Autodesk Inventor part; units mm, degrees
ref_plane "YZ Plane" through (0, 0, 0) normal (1, 0, 0) x (0, 1, 0)
ref_plane "XZ Plane" through (0, 0, 0) normal (0, 1, 0) x (-1, 0, 0)
ref_plane "XY Plane" through (0, 0, 0) normal (0, 0, 1) x (1, 0, 0)
sketch "Sketch1" plane through (0, 0, 0) normal (0, 1, 0) x (-1, 0, 0)
  line L0 (-9.525, -13.4747) -> (9.525, -13.4747)
  line L1 (9.525, -13.4747) -> (9.525, 13.4747)
  line L2 (9.525, 13.4747) -> (-9.525, 13.4747)
  line L3 (-9.525, 13.4747) -> (-9.525, -13.4747)
  line L4 (-9.525, -13.4747) -> (9.525, 13.4747) construction
  line L5 (9.525, -13.4747) -> (-9.525, 13.4747) construction
  point P0 (0, 0)
  dimension "d0" = 19.05
  dimension "d1" = 26.9494
extrude "Extrusion1" add sketch "Sketch1" along normal blind 26.9494
sketch "Sketch2" plane through (9.525, 0, 13.4747) normal (1, 0, 0) x (0, 0, -1)
  line L0 (26.9494, 26.9494) -> (0, 26.9494)
  line L1 (0, 26.9494) -> (26.9494, 0)
  line L2 (0, 0) -> (26.9494, 0)
  line L3 (26.9494, 0) -> (26.9494, 26.9494)
  line L4 (0, 26.9494) -> (26.9494, 26.9494)
  line L5 (0, 0) -> (0, 26.9494)
  point P0 (13.4747, 0)
extrude "Extrusion2" cut sketch "Sketch2" against normal blind 19.05 contours L3 L1 L0
sketch "Sketch3" plane through (0, 0, 0) normal (0, -1, 0) x (1, 0, 0)
  circle A0 centre (0, 0) radius 2.0193
  dimension "d6" = 4.0386
extrude "Extrusion3" cut sketch "Sketch3" against normal blind 19.05
thread "Thread1"
properties part number "STRU_011_BilletWedge" material "Aluminum 6061"
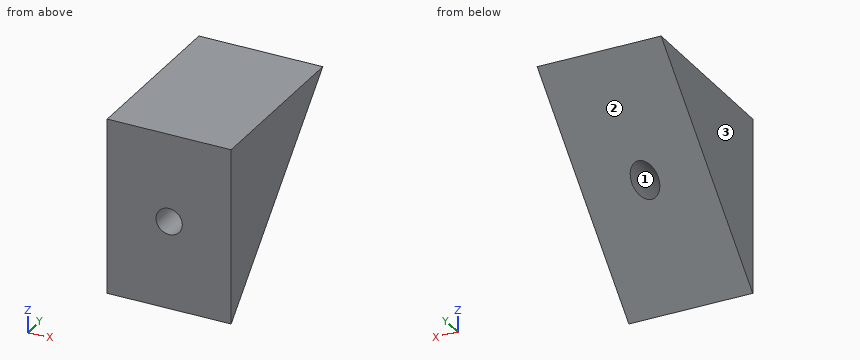
The listing builds one solid part. Answer for the finished solid, in the listing's coordinates (mm). Face numbers are marked on the shaded views. Give positions to 0.01 mm unless a question says otherwise; leave off trailing zeros. Write each loop counter-clockwise with the first axis right and the second up, starting at its lowest first coordinate (ties: lowest second). Pieces come first, ordered by that corner, then holes. Notation, with made-up numbers: (-1.5, -23) -> (27.5, -23) arc R4 ccw to (27.5, -19) -> close; hole circle Ø11 at (17, 87.25). An arc over 180 degrees is marked (long way). Use one line per item in the form item = value.
1) Section B-B on x = 0 is taken. Write down the section's boundary in (y, z).
Result:
outline = (0, -13.47) -> (11.46, -2.02) -> (0, -2.02) -> close; (0, 2.02) -> (15.49, 2.02) -> (26.95, 13.47) -> (0, 13.47) -> close
2) Section C-C on x = 5.5 is taken. Write down the section's boundary in (y, z).
Result:
outline = (0, -13.47) -> (26.95, 13.47) -> (0, 13.47) -> close
3) Section D-D on y = 14 is taken. Write down the section's boundary in (x, z) (3 decimals).
Result:
outline = (-9.525, 0.525) -> (-1.95, 0.525) arc R2.019 cw to (1.95, 0.525) -> (9.525, 0.525) -> (9.525, 13.475) -> (-9.525, 13.475) -> close
4) Section A-A on z = 0 is taken. Write down the section's boundary in (x, y) (3 decimals).
Result:
outline = (-9.525, 0) -> (-2.019, 0) -> (-2.019, 13.475) -> (-9.525, 13.475) -> close; (2.019, 0) -> (9.525, 0) -> (9.525, 13.475) -> (2.019, 13.475) -> close
5) For a pull along X with two mould halves and no side action, classify the marked faces 1, 2 and 3 as +X half, -X half, draft (parallel to the pull), parting line (faces both ways), or undercut.
Result:
face_1 = undercut
face_2 = draft
face_3 = -X half
6) Straight lines are drawn through the part: probe 1 along X at (y, z) = (7.5, 0) (3 decimals); probe 2 along Z at (x, y) = (0, 4); probe 3 along Z at (x, y) = (0, 10). For each, find the intervals that lie inside material, in ascending order.
Result:
probe_1 = -9.525 to -2.019, 2.019 to 9.525
probe_2 = -9.47 to -2.02, 2.02 to 13.47
probe_3 = -3.47 to -2.02, 2.02 to 13.47
7) Each of these flat-tipped pins is pushed along its axis until it touches: P1, Ø3, axis at x = 0, z = 0, coming from the -Y side; P2, Ø4, axis at x = -7, y = 5.5, coming from the -Z side; P3, Ø5, axis at x = -7.5, z = 2, coming from the +Y side; P4, Ø4, axis at x = 5, z = 4, coming from the +Y side. Where does it stop, or does it pass through?
Result:
P1 = through
P2 = -9.97
P3 = 17.97
P4 = 19.47
